Read the model definition and answer for the solid it produces. Units are mm, in the model's axes. Coordinates: 2 decimals unless noted, no trailing zeros. Write each loop counter-clockwise with the first axis right and the second up, starting at its lowest first coordinate (ties: lowest second). Pieces come first, ordered by that corner, then holes. Notation, with made-up numbers: (59, -0.75) -> (73, -0.75) arc R19 cw to (73, 3.25) -> close; hole circle Ø7 at (-17.5, -17). An arc over 180 degrees is marked (long way). Answer as a JSON object with one key per item and string values. Group by question number.
(1) Straight lines are drawn through the part: L1, parallel to Y at x = 15, z = 2.4; L2, parallel to Y at x = 51, z = 1.6; L3, parallel to Y at x = 61.5, z = 2.05. For each, find the intervals that lie inside material, in ascending order.
(2) Find section C-C (x = 22). Give the vertices of the cut face in (y, z), then the cut area to 3 significant figures.
(3) Flat-ended cylindrical pins translate along their axes: P1, Ø1, axis at x = 17.5, z = 1.5, coming from the -Y side; P2, Ø1.3, axis at x = 38.5, z = 1, coming from the +Y side. Find the tip coordinate at first contact, or state that the pin passes through.
(4) Find section A-A (x = 3). Give the vertices of the cut face in (y, z).
(5) Find section B-B (y = -88). Give the vertices of the cut face in (x, z).
(6) For a pull along X with two mould halves and no side action, classify faces 1 (the face through (31, -87, 2.54)), 2 (the face through (61.948, 3.608, 1.252)) as +X half, -X half, draft (parallel to the pull), parting line (faces both ways), or undercut.
(7) Find section D-D (z = 1.7). Count the separate pieces of the cut face and the enclosed holes in it, then the cut area to 3 significant figures.
from build123d import *

# Parameters (mm, degrees)
SKETCH1_R               = 2.3495
SKETCH1_R_2             = 4.445
BOSS_EXTRUDE1_DEPTH     = 2.54
SKETCH2_R               = 2.413
CUT_EXTRUDE1_DEPTH      = 217.884748371
SKETCH3_W               = 13.08488816
SKETCH3_H               = 31.623
CUT_EXTRUDE2_DEPTH      = 217.884748371
SKETCH4_W               = 12.77569874
SKETCH4_H               = 24.435209008
SKETCH4_W_2             = 40.233428475
SKETCH4_H_2             = 28.333759116
CUT_EXTRUDE3_DEPTH      = 217.884748371
SKETCH5_R               = 2.413
CUT_EXTRUDE4_DEPTH      = 217.884748371
CUT_EXTRUDE5_DEPTH      = 217.884748371
CUT_EXTRUDE5_DEPTH_BACK = 217.884748371
SKETCH8_R               = 2.3495
CUT_EXTRUDE6_DEPTH      = 191.226610272
FILLET1_R               = 1.5875
SKETCH9_W               = 0.38488816
SKETCH9_H               = 2.54
CUT_EXTRUDE7_DEPTH      = 152.146866512


with BuildPart() as part:
    # Sketch1 → Boss-Extrude1 (new body)
    with BuildSketch(Plane.XY):
        Polygon((-2.930050059, -104.509781075), (-3.314938219, -104.509781075), (-3.314938219, -110.859781075), (-3.314938219, -123.559781075), (-2.930050059, -123.559781075), (-2.930050059, -168.708281075), (38.709428475, -168.708281075), (38.709428475, -189.536281075), (105.397061781, -189.536281075), (66.517436481, -110.859781075), (45.329949941, -110.859781075), (45.329949941, -104.509781075), (45.329949941, -72.886781075), (45.329949941, -66.536781075), (66.517436481, -66.536781075), (105.397061781, 12.139718925), (38.709428475, 12.139718925), (38.709428475, -8.688281075), (-2.930050059, -8.688281075), (-2.930050059, -53.836781075), (-3.314938219, -53.836781075), (-3.314938219, -66.536781075), (-3.314938219, -72.886781075), (-2.930050059, -72.886781075), align=None)
        with Locations((90.673911143, 2.614718925)):
            Circle(SKETCH1_R, mode=Mode.SUBTRACT)
        with Locations((41.95655448, -16.435281075)):
            Circle(SKETCH1_R, mode=Mode.SUBTRACT)
        with Locations((3.035061781, -60.186781075)):
            Circle(SKETCH1_R, mode=Mode.SUBTRACT)
        with Locations((3.035061781, -117.209781075)):
            Circle(SKETCH1_R, mode=Mode.SUBTRACT)
        with Locations((41.95655448, -160.961281075)):
            Circle(SKETCH1_R, mode=Mode.SUBTRACT)
        with Locations((90.673911143, -180.011281075)):
            Circle(SKETCH1_R, mode=Mode.SUBTRACT)
        with Locations((51.409428475, -3.100281075)):
            Circle(SKETCH1_R_2, mode=Mode.SUBTRACT)
    extrude(amount=BOSS_EXTRUDE1_DEPTH)

    # Sketch2 → Cut-Extrude1 (cut, through all)
    with BuildSketch(Plane.XY.offset(2.54)):
        with Locations((13.195061781, -66.536781075)):
            Circle(SKETCH2_R)
        with Locations((34.785061781, -66.536781075)):
            Circle(SKETCH2_R)
        with Locations(Location((34.785061781, -110.859781075, 0), (0, 0, 180))):
            Circle(SKETCH2_R)
        with Locations(Location((13.195061781, -110.859781075, 0), (0, 0, 180))):
            Circle(SKETCH2_R)
    extrude(amount=-CUT_EXTRUDE1_DEPTH, mode=Mode.SUBTRACT)

    # Sketch3 → Cut-Extrude2 (cut, through all)
    with BuildSketch(Plane.XY.offset(2.54)):
        with Locations((38.787505861, -88.698281075)):
            Rectangle(SKETCH3_W, SKETCH3_H)
    extrude(amount=-CUT_EXTRUDE2_DEPTH, mode=Mode.SUBTRACT)

    # Sketch4 → Cut-Extrude3 (cut, through all)
    with BuildSketch(Plane.XY.offset(2.54)):
        with Locations((33.845579105, 3.529323429)):
            Rectangle(SKETCH4_W, SKETCH4_H)
        with Locations((20.116714238, -182.875160633)):
            Rectangle(SKETCH4_W_2, SKETCH4_H_2)
    extrude(amount=-CUT_EXTRUDE3_DEPTH, mode=Mode.SUBTRACT)

    # Sketch5 → Cut-Extrude4 (cut, through all)
    with BuildSketch(Plane(origin=(0, 0, 0), x_dir=(-1, 0, 0), z_dir=(0, 0, -1))):
        with Locations((-32.121949941, -22.404281075)):
            Circle(SKETCH5_R)
        with Locations((-32.121949941, -56.694281075)):
            Circle(SKETCH5_R)
    extrude(amount=-CUT_EXTRUDE4_DEPTH, mode=Mode.SUBTRACT)

    # Sketch7 → Cut-Extrude5 (cut, two sides: drawn at the far end of the back side and taken through both)
    with BuildSketch(Plane.XY.offset(2.54).offset(-CUT_EXTRUDE5_DEPTH_BACK)):
        Polygon((66.517436481, -66.536781075), (66.517436481, 21.52212206), (127.820808625, 21.52212206), (115.78217236, -200.256310461), (66.517436481, -200.256310461), (66.517436481, -110.859781075), align=None)
    extrude(amount=CUT_EXTRUDE5_DEPTH + CUT_EXTRUDE5_DEPTH_BACK, mode=Mode.SUBTRACT)

    # Sketch8 → Cut-Extrude6 (cut, through all)
    with BuildSketch(Plane(origin=(13.551580143, -170.546705634, 0), x_dir=(0.9999106684671756, -0.013366191885727564, 0), z_dir=(0, 0, -1))):
        with Locations(Location((44.353535624, -173.175566882, 0), (0, 0, 179.234150812))):
            Circle(SKETCH8_R)
        with Locations(Location((46.68181957, 8.1642617, 0), (0, 0, 179.234150812))):
            Circle(SKETCH8_R)
    extrude(amount=-CUT_EXTRUDE6_DEPTH, mode=Mode.SUBTRACT)

    # Fillet1
    fillet1_edges = [part.edges().sort_by_distance(p)[0] for p in [
        (45.329949941, -72.886781075, 1.27),
        (45.329949941, -104.509781075, 1.27),
        (32.245061781, -104.509781075, 1.27),
        (32.245061781, -72.886781075, 1.27),
        (40.233428475, -189.536281075, 1.27),
        (40.233428475, 12.139718925, 1.27),
        (40.233428475, -8.688281075, 1.27),
        (40.233428475, -168.708281075, 1.27),
        (66.517436481, 12.139718925, 1.27),
        (66.517436481, -189.536281075, 1.27),
        (45.329949941, -66.536781075, 1.27),
        (45.329949941, -110.859781075, 1.27),
        (66.517436481, -110.859781075, 1.27),
        (-2.930050059, -168.708281075, 1.27),
        (-2.930050059, -8.688281075, 1.27),
        (66.517436481, -66.536781075, 1.27),
    ]]
    fillet(fillet1_edges, radius=FILLET1_R)

    # Sketch9 → Cut-Extrude7 (cut, through all)
    with BuildSketch(Plane.XZ.offset(123.559781075)):
        with Locations((-3.122494139, 1.27)):
            Rectangle(SKETCH9_W, SKETCH9_H)
    extrude(amount=-CUT_EXTRUDE7_DEPTH, mode=Mode.SUBTRACT)


solid = part.part
Results below:
{
 "1": {"L1": "y = -168.71 to -112.46, -109.26 to -68.14, -64.94 to -8.69", "L2": "y = -189.54 to -110.86, -66.54 to -7.53, 1.33 to 12.14", "L3": "y = -189.54 to -181.24, -177.43 to -110.86, -66.54 to 0.05, 3.99 to 12.14"},
 "2": {"outline": "(-168.71, 0) -> (-8.69, 0) -> (-8.69, 2.54) -> (-168.71, 2.54) -> close", "area": "406 mm2"},
 "3": {"P1": "stops at y = -168.71", "P2": "stops at y = -8.61"},
 "4": {"outline": "(-168.71, 0) -> (-119.56, 0) -> (-119.56, 2.54) -> (-168.71, 2.54) -> close; (-114.86, 0) -> (-62.54, 0) -> (-62.54, 2.54) -> (-114.86, 2.54) -> close; (-57.84, 0) -> (-8.69, 0) -> (-8.69, 2.54) -> (-57.84, 2.54) -> close"},
 "5": {"outline": "(-2.93, 0) -> (32.25, 0) -> (32.25, 2.54) -> (-2.93, 2.54) -> close"},
 "6": {"face 1": "draft", "face 2": "undercut"},
 "7": {"separate pieces": "1", "enclosed holes": "13", "area": "10,600 mm2"}
}
